from build123d import *
from OCP.BRepFilletAPI import BRepFilletAPI_MakeChamfer

# Parameters (mm, degrees)
EXTRUDE_1_DEPTH     = 3
SKETCH_2_R          = 5
SKETCH_2_R_2        = 1.25
CUT_EXTRUDE_1_DEPTH = 95.288122264
CUT_EXTRUDE_2_DEPTH = 1.6
SKETCH_4_R          = 2
SKETCH_4_R_2        = 1.25
EXTRUDE_2_DEPTH     = 2
CHAMFER_1_SIZE      = 0.5
CHAMFER_1_SIZE2     = 0.288675135


with BuildPart() as part:
    # 草圖1 → 填料-伸長1 (new body)
    with BuildSketch(Plane.XY):
        with BuildLine():
            Line((35.5, 33), (35.5, 29))
            ThreePointArc((35.5, 29), (36.085786438, 27.585786438), (37.5, 27))
            Line((37.5, 27), (85.5, 27))
            ThreePointArc((85.5, 27), (86.914213562, 26.414213562), (87.5, 25))
            Line((87.5, 25), (87.5, -25))
            ThreePointArc((87.5, -25), (86.914213562, -26.414213562), (85.5, -27))
            Line((85.5, -27), (37.5, -27))
            ThreePointArc((37.5, -27), (36.085786438, -27.585786438), (35.5, -29))
            Line((35.5, -29), (35.5, -33))
            ThreePointArc((35.5, -33), (34.914213562, -34.414213562), (33.5, -35))
            Line((33.5, -35), (-33.5, -35))
            ThreePointArc((-33.5, -35), (-34.914213562, -34.414213562), (-35.5, -33))
            Line((-35.5, -33), (-35.5, -29))
            ThreePointArc((-35.5, -29), (-36.085786438, -27.585786438), (-37.5, -27))
            Line((-37.5, -27), (-85.5, -27))
            ThreePointArc((-85.5, -27), (-86.914213562, -26.414213562), (-87.5, -25))
            Line((-87.5, -25), (-87.5, 25))
            ThreePointArc((-87.5, 25), (-86.914213562, 26.414213562), (-85.5, 27))
            Line((-85.5, 27), (-37.5, 27))
            ThreePointArc((-37.5, 27), (-36.085786438, 27.585786438), (-35.5, 29))
            Line((-35.5, 29), (-35.5, 33))
            ThreePointArc((-35.5, 33), (-34.914213562, 34.414213562), (-33.5, 35))
            Line((-33.5, 35), (33.5, 35))
            ThreePointArc((33.5, 35), (34.914213562, 34.414213562), (35.5, 33))
        make_face()
    extrude(amount=EXTRUDE_1_DEPTH)

    # 草圖2 → 除料-伸長1 (cut, through all)
    with BuildSketch(Plane.XY.offset(3)):
        Circle(SKETCH_2_R)
        with Locations((27, -13.5)):
            Circle(SKETCH_2_R_2)
        with Locations((6, -13.5)):
            Circle(SKETCH_2_R_2)
        with Locations((6, -26)):
            Circle(SKETCH_2_R_2)
        with Locations((27, -26)):
            Circle(SKETCH_2_R_2)
        with BuildLine():
            Line((43.5, -22.5), (43.5, 22.5))
            ThreePointArc((43.5, 22.5), (45, 24), (46.5, 22.5))
            Line((46.5, 22.5), (46.5, -22.5))
            ThreePointArc((46.5, -22.5), (45, -24), (43.5, -22.5))
        make_face()
        with BuildLine():
            Line((-46.5, -22.5), (-46.5, 22.5))
            ThreePointArc((-46.5, 22.5), (-45, 24), (-43.5, 22.5))
            Line((-43.5, 22.5), (-43.5, -22.5))
            ThreePointArc((-43.5, -22.5), (-45, -24), (-46.5, -22.5))
        make_face()
        with BuildLine():
            Line((-82.5, -22.5), (-82.5, 22.5))
            ThreePointArc((-82.5, 22.5), (-81, 24), (-79.5, 22.5))
            Line((-79.5, 22.5), (-79.5, -22.5))
            ThreePointArc((-79.5, -22.5), (-81, -24), (-82.5, -22.5))
        make_face()
        with BuildLine():
            Line((79.5, -22.5), (79.5, 22.5))
            ThreePointArc((79.5, 22.5), (81, 24), (82.5, 22.5))
            Line((82.5, 22.5), (82.5, -22.5))
            ThreePointArc((82.5, -22.5), (81, -24), (79.5, -22.5))
        make_face()
        with BuildLine():
            Line((21.5, -31.5), (8.5, -31.5))
            ThreePointArc((8.5, -31.5), (7, -30), (8.5, -28.5))
            Line((8.5, -28.5), (21.5, -28.5))
            ThreePointArc((21.5, -28.5), (23, -30), (21.5, -31.5))
        make_face()
        with BuildLine():
            Line((-21.5, -31.5), (-8.5, -31.5))
            ThreePointArc((-8.5, -31.5), (-7, -30), (-8.5, -28.5))
            Line((-8.5, -28.5), (-21.5, -28.5))
            ThreePointArc((-21.5, -28.5), (-23, -30), (-21.5, -31.5))
        make_face()
        with BuildLine():
            Line((21.5, 31.5), (8.5, 31.5))
            ThreePointArc((8.5, 31.5), (7, 30), (8.5, 28.5))
            Line((8.5, 28.5), (21.5, 28.5))
            ThreePointArc((21.5, 28.5), (23, 30), (21.5, 31.5))
        make_face()
        with BuildLine():
            Line((-21.5, 31.5), (-8.5, 31.5))
            ThreePointArc((-8.5, 31.5), (-7, 30), (-8.5, 28.5))
            Line((-8.5, 28.5), (-21.5, 28.5))
            ThreePointArc((-21.5, 28.5), (-23, 30), (-21.5, 31.5))
        make_face()
        with BuildLine():
            Line((21.5, 24), (8.5, 24))
            ThreePointArc((8.5, 24), (7, 22.5), (8.5, 21))
            Line((8.5, 21), (21.5, 21))
            ThreePointArc((21.5, 21), (23, 22.5), (21.5, 24))
        make_face()
        with BuildLine():
            Line((-21.5, 24), (-8.5, 24))
            ThreePointArc((-8.5, 24), (-7, 22.5), (-8.5, 21))
            Line((-8.5, 21), (-21.5, 21))
            ThreePointArc((-21.5, 21), (-23, 22.5), (-21.5, 24))
        make_face()
        with BuildLine():
            Line((-21.5, -24), (-8.5, -24))
            ThreePointArc((-8.5, -24), (-7, -22.5), (-8.5, -21))
            Line((-8.5, -21), (-21.5, -21))
            ThreePointArc((-21.5, -21), (-23, -22.5), (-21.5, -24))
        make_face()
        with BuildLine():
            Line((21.5, -24), (8.5, -24))
            ThreePointArc((8.5, -24), (7, -22.5), (8.5, -21))
            Line((8.5, -21), (21.5, -21))
            ThreePointArc((21.5, -21), (23, -22.5), (21.5, -24))
        make_face()
    extrude(amount=-CUT_EXTRUDE_1_DEPTH, mode=Mode.SUBTRACT)

    # 草圖3 → 除料-伸長2 (cut)
    with BuildSketch(Plane.XY.offset(3)):
        Polygon((29.309401077, -26), (28.154700538, -24), (25.845299462, -24), (24.690598923, -26), (25.845299462, -28), (28.154700538, -28), align=None)
        Polygon((8.309401077, -26), (7.154700538, -24), (4.845299462, -24), (3.690598923, -26), (4.845299462, -28), (7.154700538, -28), align=None)
        Polygon((29.309401077, -13.5), (28.154700538, -11.5), (25.845299462, -11.5), (24.690598923, -13.5), (25.845299462, -15.5), (28.154700538, -15.5), align=None)
        Polygon((8.309401077, -13.5), (7.154700538, -11.5), (4.845299462, -11.5), (3.690598923, -13.5), (4.845299462, -15.5), (7.154700538, -15.5), align=None)
    extrude(amount=-CUT_EXTRUDE_2_DEPTH, mode=Mode.SUBTRACT)

    # 草圖4 → 填料-伸長2 (add)
    # profile 1 of 4: a face of its own
    with BuildSketch(Plane(origin=(0, 0, 0), x_dir=(-1, 0, 0), z_dir=(0, 0, -1))):
        with Locations(Location((-27, -13.5, 0), (0, 0, 180))):
            Circle(SKETCH_4_R)
        with Locations(Location((-27, -13.5, 0), (0, 0, 180))):
            Circle(SKETCH_4_R_2, mode=Mode.SUBTRACT)
    # profile 2 of 4: a face of its own
    with BuildSketch(Plane(origin=(0, 0, 0), x_dir=(-1, 0, 0), z_dir=(0, 0, -1))):
        with Locations(Location((-27, -26, 0), (0, 0, 180))):
            Circle(SKETCH_4_R)
        with Locations(Location((-27, -26, 0), (0, 0, 180))):
            Circle(SKETCH_4_R_2, mode=Mode.SUBTRACT)
    # profile 3 of 4: a face of its own
    with BuildSketch(Plane(origin=(0, 0, 0), x_dir=(-1, 0, 0), z_dir=(0, 0, -1))):
        with Locations(Location((-6, -13.5, 0), (0, 0, 180))):
            Circle(SKETCH_4_R)
        with Locations(Location((-6, -13.5, 0), (0, 0, 180))):
            Circle(SKETCH_4_R_2, mode=Mode.SUBTRACT)
    # profile 4 of 4: a face of its own
    with BuildSketch(Plane(origin=(0, 0, 0), x_dir=(-1, 0, 0), z_dir=(0, 0, -1))):
        with Locations(Location((-6, -26, 0), (0, 0, 180))):
            Circle(SKETCH_4_R)
        with Locations(Location((-6, -26, 0), (0, 0, 180))):
            Circle(SKETCH_4_R_2, mode=Mode.SUBTRACT)
    extrude(amount=EXTRUDE_2_DEPTH)

    # 導角1: one chamfer whose edges measure the first distance from different faces: ONE call of the kernel's chamfer builder (chamfer() names one face for all edges)
    chamfer_1_edges_1 = [part.edges().sort_by_distance(p)[0] for p in [
        (25.75, -13.5, -2),
    ]]
    chamfer_1_side_1 = [part.faces().sort_by_distance(p)[0] for p in [
        (25.056568542, -13.5, -2),
    ]]
    chamfer_1_edges_2 = [part.edges().sort_by_distance(p)[0] for p in [
        (25.75, -26, -2),
    ]]
    chamfer_1_side_2 = [part.faces().sort_by_distance(p)[0] for p in [
        (25.056568542, -26, -2),
    ]]
    chamfer_1_edges_3 = [part.edges().sort_by_distance(p)[0] for p in [
        (4.75, -13.5, -2),
    ]]
    chamfer_1_side_3 = [part.faces().sort_by_distance(p)[0] for p in [
        (4.056568542, -13.5, -2),
    ]]
    chamfer_1_edges_4 = [part.edges().sort_by_distance(p)[0] for p in [
        (4.75, -26, -2),
    ]]
    chamfer_1_side_4 = [part.faces().sort_by_distance(p)[0] for p in [
        (4.056568542, -26, -2),
    ]]
    chamfer_1 = BRepFilletAPI_MakeChamfer(part.part.solid().wrapped)
    for e in chamfer_1_edges_1:
        chamfer_1.Add(CHAMFER_1_SIZE, CHAMFER_1_SIZE2, e.wrapped, chamfer_1_side_1[0].wrapped)  # the first distance lies on this face
    for e in chamfer_1_edges_2:
        chamfer_1.Add(CHAMFER_1_SIZE, CHAMFER_1_SIZE2, e.wrapped, chamfer_1_side_2[0].wrapped)  # the first distance lies on this face
    for e in chamfer_1_edges_3:
        chamfer_1.Add(CHAMFER_1_SIZE, CHAMFER_1_SIZE2, e.wrapped, chamfer_1_side_3[0].wrapped)  # the first distance lies on this face
    for e in chamfer_1_edges_4:
        chamfer_1.Add(CHAMFER_1_SIZE, CHAMFER_1_SIZE2, e.wrapped, chamfer_1_side_4[0].wrapped)  # the first distance lies on this face
    add(Compound.cast(chamfer_1.Shape()), mode=Mode.REPLACE)


solid = part.part
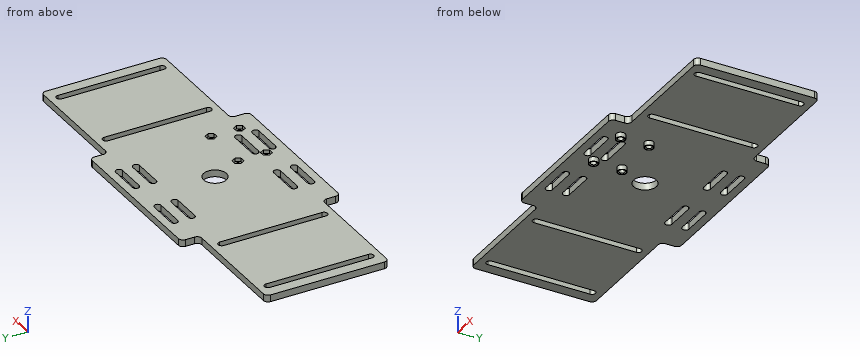
Read the model definition and answer for the solid it produces. Units are mm, in the model's axes. Coordinates: 2 decimals unless noted, no trailing zeros. Loops run counter-clockwise (first coordinate to the right, second up) from the corner with the lowest first, then second, coordinate; pieces in that order, holes last. Notation, with made-up numbers: (36.25, -35.75) -> (75.25, -35.75) arc R14 cw to (75.25, -15.75) -> close; hole circle Ø1 at (55, -7.5). An arc over 180 degrees is marked (long way). Answer in a Markdown table with one row per item.
Item 1: Each of these flat-tipped pins is pushed along its axis until it touches: P1, Ø3, axis at x = 61, z = 2.5, coming from the -Y side; P2, Ø2.5, axis at y = 31, z = 1, coming from the -X side; P3, Ø4, axis at x = -48, y = 8, coming from the -Z side; P4, Ø3, axis at x = 26.5, y = -12.5, coming from the +Z side. Where does it stop, or does it pass through?
Returned:
| item | result |
|---|---|
| P1 | stops at y = -27 |
| P2 | stops at x = -35.5 |
| P3 | stops at z = 0 |
| P4 | stops at z = 3 |
Item 2: A cutting plane is placed at A-A on y = -7.5. Determine the outline of the cut face in (x, z), plus the area to 3 significant figures.
Returned:
| item | result |
|---|---|
| outline | (-87.5, 0) -> (-82.5, 0) -> (-82.5, 3) -> (-87.5, 3) -> close; (-79.5, 0) -> (-46.5, 0) -> (-46.5, 3) -> (-79.5, 3) -> close; (-43.5, 0) -> (43.5, 0) -> (43.5, 3) -> (-43.5, 3) -> close; (46.5, 0) -> (79.5, 0) -> (79.5, 3) -> (46.5, 3) -> close; (82.5, 0) -> (87.5, 0) -> (87.5, 3) -> (82.5, 3) -> close |
| area | 489 mm^2 |
Item 3: A cutting plane is placed at C-C on z = 2.2. Give the number of separate pieces and of enclosed holes in the cut face, plus the area to 3 significant figures.
Returned:
| item | result |
|---|---|
| separate pieces | 1 |
| enclosed holes | 17 |
| area | 9,510 mm^2 |
Item 4: A cutting plane is placed at B-B on y = 0. Determine the outline of the cut face in (x, z), plus the area to 3 significant figures.
Returned:
| item | result |
|---|---|
| outline | (-87.5, 0) -> (-82.5, 0) -> (-82.5, 3) -> (-87.5, 3) -> close; (-79.5, 0) -> (-46.5, 0) -> (-46.5, 3) -> (-79.5, 3) -> close; (-43.5, 0) -> (-5, 0) -> (-5, 3) -> (-43.5, 3) -> close; (5, 0) -> (43.5, 0) -> (43.5, 3) -> (5, 3) -> close; (46.5, 0) -> (79.5, 0) -> (79.5, 3) -> (46.5, 3) -> close; (82.5, 0) -> (87.5, 0) -> (87.5, 3) -> (82.5, 3) -> close |
| area | 459 mm^2 |
Item 5: Straight lines are drawn through the part: line 1 along Y through (x, z) = (6, -0.65); line 2 along Y through (x, z) = (9.5, 2.65); line 3 along X through (y, z) = (-8, 0.75). For each, find the intervals that lie inside material, in ascending order. Write a range as [from, to].
Returned:
| item | result |
|---|---|
| line 1 | y = [-28, -27.25], [-24.75, -24], [-15.5, -14.75], [-12.25, -11.5] |
| line 2 | y = [-35, -31.5], [-28.5, -24], [-21, 21], [24, 28.5], [31.5, 35] |
| line 3 | x = [-87.5, -82.5], [-79.5, -46.5], [-43.5, 43.5], [46.5, 79.5], [82.5, 87.5] |
